Autodesk Inventor part; units mm, degrees
ref_plane "YZ Plane" through (0, 0, 0) normal (1, 0, 0) x (0, 1, 0)
ref_plane "XZ Plane" through (0, 0, 0) normal (0, 1, 0) x (-1, 0, 0)
ref_plane "XY Plane" through (0, 0, 0) normal (0, 0, 1) x (1, 0, 0)
sketch "Sketch1" plane through (0, 0, 0) normal (0, 0, 1) x (1, 0, 0)
  line L0 (0, 0) -> (38.1, 0)
  line L1 (38.1, 0) -> (48.2818, -36.7143)
  line L2 (38.1, 0) -> (76.2, 0) construction
  line L3 (45.343, 9.525) -> (9.525, 9.525)
  line L4 (0, 0) -> (0, 17.78)
  line L5 (0, 17.78) -> (9.525, 17.78)
  line L6 (9.525, 17.78) -> (9.525, 9.525)
  line L7 (0, 9.525) -> (9.525, 9.525)
  line L8 (45.343, 9.525) -> (38.1, 0)
  line L9 (48.2818, -36.7143) -> (66.6389, -31.6234)
  line L10 (66.6389, -31.6234) -> (64.0935, -22.4448)
  line L11 (64.0935, -22.4448) -> (54.9149, -24.9903)
  line L12 (54.9149, -24.9903) -> (45.343, 9.525)
  dimension "d0" = 38.1
  dimension "d1" = 38.1
  dimension "d2" = 74.5
  dimension "d9" = 17.78
  dimension "d10" = 9.525
  dimension "d11" = 9.525
  dimension "d12" = 19.05
  dimension "d13" = 9.525
  dimension "d14" = 9.525
extrude "Extrusion1" add sketch "Sketch1" along normal blind 10.16
properties part number "AttachmentPlateHopper_v2"
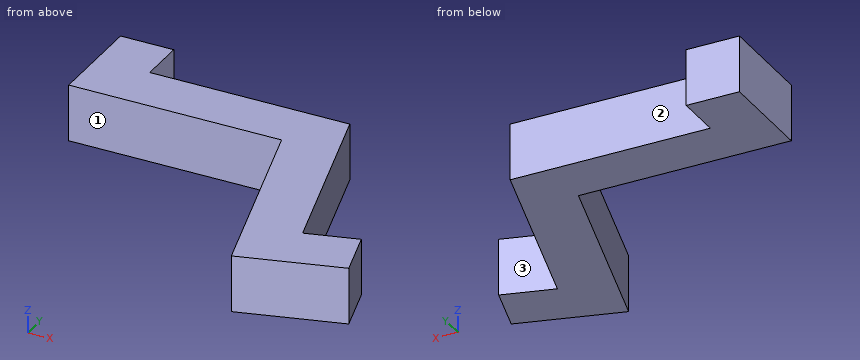
Model file for the job. Use its own axes, mm. Face numbers are marked on the shaded views. A direction names the side the tool comes from. Round coordinates to 2 decimals unless told otherwise and drop trailing zeros. Write each loop counter-clockwise with the first axis right and the second up, starting at its lowest first coordinate (ties: lowest second). Pieces come first, ordered by that corner, then holes. Notation, with made-up numbers: (15, 17.25) - (62, 17.25) arc R17 cw to (62, 33.25) - close; hole circle Ø7 at (37, 11). An arc over 180 degrees is marked (long way). One line per item, written item: value.
(1) Cut at A-A, the plane z = 3. Give the cut face in (x, y) (1 decimal).
Values follow:
outline: (0, 0) - (38.1, 0) - (48.3, -36.7) - (66.6, -31.6) - (64.1, -22.4) - (54.9, -25) - (45.3, 9.5) - (9.5, 9.5) - (9.5, 17.8) - (0, 17.8) - close
(2) Cut at C-C, the plane x = 6. Give the cut face in (y, z), plus the area to 3 significant figures.
Values follow:
outline: (0, 0) - (17.78, 0) - (17.78, 10.16) - (0, 10.16) - close
area: 181 mm²
(3) Cut at B-B, the plane y = 12. Give the cut face in (x, z) (3 decimals), plus the area to 3 significant figures.
Values follow:
outline: (0, 0) - (9.525, 0) - (9.525, 10.16) - (0, 10.16) - close
area: 96.8 mm²
(4) Wall check: probe 1 along Y at (x, z) = (21, 7.75) (3 decimals); probe 2 along Y at (x, z) = (9, 9.25); probe 3 along X at (y, z) = (5.5, 7). Give the ranges that are in metal, low to high.
Values follow:
probe 1: y = 0 to 9.525
probe 2: y = 0 to 17.78
probe 3: x = 0 to 46.46
(5) 3-axis set-ups, long thin cutter, end or side, ignore diameter. For the marked faces 1, 2 and 3: which of +Z, -Z, +X, -X, +Y, -Y reach the whole face in a straight line?
Values follow:
face 1: +Z, -Z, -X, -Y
face 2: +Z, -Z, +X, +Y
face 3: +Z, -Z, +Y
(6) Drop flat-ended pins along their axis: P1, Ø1.5, axis at x = 29.5, z = 6, coming from the +Y side (3 decimals); P2, Ø6, axis at x = 15, z = 7.5, coming from the -Y side; P3, Ø1, axis at y = 6.5, z = 5.5, coming from the +X side. Give the stop position or say it passes through.
Values follow:
P1: stops at y = 9.525
P2: stops at y = 0
P3: stops at x = 46.32
